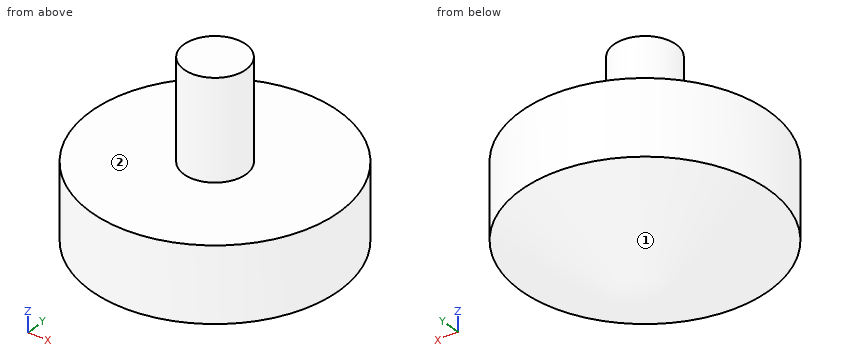
```python
from build123d import *

# Parameters (mm, degrees)
F0_R     = 12.7
F1_DEPTH = 15.24
F2_SIZE2 = 12.7
F2_SIZE  = 7.62
F4_R     = 3.175
F5_R     = 3.175


with BuildPart() as f1:
    # F0 (on Top) → F1 (new body)
    with BuildSketch(Plane.XY):
        with Locations((-52.3585453629, 15.3619199991)):
            Circle(F0_R)
    extrude(amount=F1_DEPTH)

    # F2
    f2_edges = [f1.edges().sort_by_distance(p)[0] for p in [
        (-65.058545, 15.36192, 0),
    ]]
    f2_side = f1.faces().sort_by_distance((-65.058545, 15.36192, 7.62))[0]
    chamfer(f2_edges, length=F2_SIZE, length2=F2_SIZE2, reference=f2_side)

    # F4 (on face) → F6 section 0
    with BuildSketch(Plane.XY.offset(15.24)):
        with Locations((-52.3585453629, 15.3619199991)):
            Circle(F4_R)
    # F5 (on offset) → F6 section 1
    with BuildSketch(Plane.XY.offset(25.4)):
        with Locations((-52.3585453629, 15.3619199991)):
            Circle(F5_R)
    loft()


solid = f1.part
```
The listing builds one solid part. Answer for the finished solid, in the listing's coordinates (mm). Face numbers are marked on the shaded views. A direction names the side the tool comes from. Coordinates: 2 decimals unless noted, no trailing zeros. Loops run counter-clockwise (first coordinate to the right, second up) from the corner with the lowest first, then second, coordinate; pieces in that order, holes last. Notation, with made-up numbers: (-36, 38) - (9, 38) arc R27 cw to (9, 64) - close; hole circle Ø3 at (60.25, -37.75). An arc over 180 degrees is marked (long way). Use a Markdown table: item, result. Add a question column.
1) For the marked faces 1 and 2, determine the directions among +Z, -Z, +X, -X, +Y, -Y from which every point of the face is accessible in a straight line to the end or side of a thin tool.
2) The part is cut by section A-A, the plane z = 23. Give the vertices of the cut face in (x, y) (3 decimals), and give its area (3 significant figures).
3) Given pin 1 (2 mm diameter, centred on x = -43.5, y = 17, fed in from -Z); pin 2 (10 mm diameter, centred on y = 6, z = 16.5, fed in from +X); pin 3 (6 mm diameter, centred on y = 10.5, z = 7, fed in from +X); pin 4 (3 mm diameter, centred on y = 8.5, z = 17.5, fed in from +X), each flat-ended and moving along its own axis, determine where each tip first touches the part or whether it passes through.
4) Find the intervals of material crossed by line 1 (Y direction, x = -53.5, z = 23.75); line 2 (Z direction, x = -60.5, y = 9.5); line 3 (Z direction, x = -47.25, y = 11), in increasing order.
5) The part is cut by section B-B, the plane z = 7.25. Give the vertices of the cut face in (x, y), and give its area (3 significant figures).
Here are the results:
| question | item | result |
|---|---|---|
| 1 | face 1 | -Z |
| 1 | face 2 | +Z |
| 2 | outline | circle Ø6.35 at (-52.359, 15.362) |
| 2 | area | 31.7 mm^2 |
| 3 | pin 1 | stops at z = 4.81 |
| 3 | pin 2 | stops at x = -40.49 |
| 3 | pin 3 | stops at x = -39.81 |
| 3 | pin 4 | passes through |
| 4 | line 1 | y = 12.4 to 18.32 |
| 4 | line 2 | z = 6.02 to 15.24 |
| 4 | line 3 | z = 4.03 to 15.24 |
| 5 | outline | circle Ø24.17 at (-52.36, 15.36) |
| 5 | area | 459 mm^2 |
